Design review of the part built by this model. Coordinates are the model's own, in mm. A direction names the side the tool comes from. Round coordinates to 2 decimals unless told otherwise and drop trailing zeros. Write each loop counter-clockwise with the first axis right and the second up, starting at its lowest first coordinate (ties: lowest second). Pieces come first, ordered by that corner, then holes. Notation, with made-up numbers: (-18, -11.75) -> (13, -11.75) arc R21 cw to (13, 16.25) -> close; hole circle Ø7 at (84, 24). An arc over 180 degrees is marked (long way). One line per question, with ' | ' between items. Start each with the question number.
1) Insertion check: pin 1 Ø19.5 at (y, z) = (109.6, 11.94) entering from -X; pin 2 Ø19.5 at (y, z) = (-119.48, 32.13) entering from -X; pin 3 Ø6 at (y, z) = (-50, 4.5) entering from -X. Each pin has a flat end and moves straight along its axis. Give the tip position at first contact, or say it passes through.
2) For probe 1 along Y at (x, z) = (-8, 37.5); probe 2 along Y at (x, z) = (-11, 5); probe 3 along X at (y, z) = (93.5, 26), list the stretches that pass through material, from the lowest coordinate up.
3) Consider section A-A (x = -25.5). Give the boundary of the cut face in (y, z).
4) Consider section C-C (x = -49.5). Give the boundary of the cut face in (y, z), then the cut area to 3 significant figures.
5) Consider section B-B (z = 35). Give the boundary of the cut face in (x, y), then the cut area to 3 significant figures.
6) For faces 4 (the flat face through (-7, 130.068, 23)), 5 (the flat face through (-12.362, -118, 22)), 6 (the cylindrical face through (-5.55, -111.99, 32.46)), 7 (the flat face through (-13.5, 110, 23)), 8 (the flat face through (0, 108, 23)), list the 3-axis set-ups (+Z, -Z, +X, -X, +Y, -Y) from which the entire face can be reached by the end or side of a thin tool; tool diameter is ignored.
7) Consider section D-D (y = 48). Give the boundary of the cut face in (x, z).
8) Mouldability with a two-part tool opening along Y and no side actions: class faces 1 (the cylindrical face through (-6.84, 115.55, 27.57)), 2 (the flat face through (1.529, -99, 22)), 3 (the cylindrical face through (-70.49, -2.99, 22.18)) as +Y half, -Y half, draft (parallel to the pull), parting line (faces both ways), or undercut.
```python
from build123d import *

# Parameters (mm, degrees)
BOSS_EXTRUDE1_DEPTH = 45
BOSS_EXTRUDE4_DEPTH = 45
BOSS_EXTRUDE5_DEPTH = 45
SKETCH9_R           = 7.5
CUT_EXTRUDE1_DEPTH  = 42.5


with BuildPart() as part:
    # Sketch3 → Boss-Extrude1 (new body)
    with BuildSketch(Plane(origin=(0, 0, 0), x_dir=(0, 1, 0), z_dir=(0, 0, 1))):
        with BuildLine():
            Line((-104.44581982, -1.529393099), (-93.813362353, -1.529393099))
            ThreePointArc((-93.813362353, -1.529393099), (-4.955593322, 59.935089755), (84.940851468, 0))
            Line((84.940851468, 0), (95.96089631, 0))
            ThreePointArc((95.96089631, 0), (-4.786263807, 70.493362274), (-104.44581982, -1.529393099))
        make_face()
    extrude(amount=BOSS_EXTRUDE1_DEPTH)

    # Sketch7 → Boss-Extrude4 (add)
    with BuildSketch(Plane(origin=(0, 95.96089631, 45), x_dir=(1, 0, 0), z_dir=(0, 0, -1))):
        Polygon((-13.5, 5.893061873), (-13.5, -34.106938127), (0, -34.106938127), (0, 0), align=None)
    extrude(amount=BOSS_EXTRUDE4_DEPTH)

    # Sketch8 → Boss-Extrude5 (add)
    with BuildSketch(Plane(origin=(1.529393099, -104.44581982, 0), x_dir=(1, 0, 0), z_dir=(0, 0, -1))):
        Polygon((-13.891184433, -5.839173076), (-13.891184433, 34.160826924), (-0.391184433, 34.160826924), (0, 0), align=None)
    extrude(amount=-BOSS_EXTRUDE5_DEPTH)

    # Sketch9 → Cut-Extrude1 (cut, symmetric)
    with BuildSketch(Plane(origin=(-12.361791334, 0, 0), x_dir=(0, -1, 0), z_dir=(-1, 0, 0))):
        with Locations((119.481769574, 11.944393397)):
            Circle(SKETCH9_R)
        with Locations((119.481769574, 32.133475773)):
            Circle(SKETCH9_R)
        with Locations((-109.597018442, 11.944393397)):
            Circle(SKETCH9_R)
        with Locations((-109.597018442, 32.133475773)):
            Circle(SKETCH9_R)
    extrude(amount=CUT_EXTRUDE1_DEPTH, both=True, mode=Mode.SUBTRACT)


solid = part.part
```
From the geometry:
1) pin 1: stops at x = -13.5 | pin 2: stops at x = -12.36 | pin 3: stops at x = -61.38
2) probe 1: y = -138.61 to -124.72, -114.24 to -89.52, 81.25 to 104.36, 114.84 to 130.07 | probe 2: y = -138.61 to -122.31, -116.65 to -87.9, 79.63 to 106.76, 112.43 to 130.07 | probe 3: x = -13.5 to 0
3) outline: (-90.71, 0) -> (-77.87, 0) -> (-77.87, 45) -> (-90.71, 45) -> close; (69.6, 0) -> (82.75, 0) -> (82.75, 45) -> (69.6, 45) -> close
4) outline: (-67.33, 0) -> (-47.7, 0) -> (-47.7, 45) -> (-67.33, 45) -> close; (39.44, 0) -> (59.38, 0) -> (59.38, 45) -> (39.44, 45) -> close | area: 1,780 mm2
5) outline: (-13.5, 90.07) arc R106.09 ccw to (-12.36, -98.61) -> (-12.36, -112.55) -> (1.44, -112.55) -> (1.53, -104.45) -> (1.53, -93.81) arc R96.15 cw to (0, 84.94) -> (0, 102.67) -> (-13.5, 102.67) -> close; (-13.5, 116.53) -> (0, 116.53) -> (0, 130.07) -> (-13.5, 130.07) -> close; (-12.36, -138.61) -> (1.14, -138.61) -> (1.28, -126.41) -> (-12.36, -126.41) -> close | area: 3,190 mm2
6) face 4: +Z, -Z, +X, -X, +Y | face 5: +Z, -Z, -X, -Y | face 6: +X, -X | face 7: +Z, -Z, -X, +Y | face 8: +Z, -Z, +X, +Y
7) outline: (-56.89, 0) -> (-44.58, 0) -> (-44.58, 45) -> (-56.89, 45) -> close
8) face 1: undercut | face 2: draft | face 3: parting line
